from build123d import *

# Parameters (mm, degrees)
F0_W     = 25
F0_H     = 35
F1_DEPTH = 25
F3_R     = 5


with BuildPart() as f1:
    # F0 (on Top) → F1 (new body)
    with BuildSketch(Plane.XY):
        with Locations((-81.198196, -25.874247)):
            Rectangle(F0_W, F0_H)
        with Locations((-81.198196, 214.125753)):
            Rectangle(F0_W, F0_H)
        Polygon((-2.448196, 256.625753), (-68.698196, 256.625753), (-68.698196, 231.625753), (-68.698196, 196.625753), (-68.698196, -8.374247), (-68.698196, -43.374247), (-68.698196, -68.374247), (-2.448196, -68.374247), align=None)
    extrude(amount=F1_DEPTH)

    # F2: F1 across face


with BuildPart() as f1_1:
    add(f1.part)
    add(f1.part.mirror(Plane(origin=(-2.448196, 94.125753, 12.5), x_dir=(0, 1, 0), z_dir=(1, 0, 0))))

    # F3
    f3_edges = [f1_1.edges().sort_by_distance(p)[0] for p in [
        (-2.448196, 256.625753, 0),
        (-2.448196, 256.625753, 25),
        (-2.448196, -68.374247, 0),
        (-2.448196, -68.374247, 25),
    ]]
    fillet(f3_edges, radius=F3_R)


solid = f1_1.part
Design review of the part built by this model. Coordinates are the model's own, in mm. A direction names the side the tool comes from. Coordinates: 2 decimals unless noted, no trailing zeros. Order: outer loops, then holes, each group sorted by start corner. A loop starts at its lowest first (then second) coordinate and runs counter-clockwise, first axis right, second up. Notation, with made-up numbers: (-8, 34) -> (4, 34) arc R10 ccw to (4, 43) -> close; hole circle Ø7 at (-13, 6.5). An arc over 180 degrees is marked (long way). Use one line per item in the form item = value. Start each with the question number.
(1) For faces 5 (the flat face through (-68.698, 244, 12)), 6 (the flat face through (-81, 196.626, 12)), 7 (the flat face through (63.802, 96, 12)), 8 (the flat face through (-68.698, -56, 12)), list the 3-axis set-ups (+Z, -Z, +X, -X, +Y, -Y) from which the entire face can be reached by the end or side of a thin tool; tool diameter is ignored.
(2) The part is to be moulded in two halves that separate along Y. For faces 1 (the flat face through (-1, 96, 25)), 2 (the flat face through (76, -43.374, 12)), 3 (the flat face through (76, 196.626, 12)), 4 (the flat face through (-68.698, 96, 12)), say which applies: +Y half, -Y half, draft (parallel to the pull), parting line (faces both ways), or undercut.
(3) Add section B-B on y = 140. State the section outline as (x, z) points, plus the area to 3 significant figures.
(4) Add section A-A on z = 13.75. State the section outline as (x, y) points, plus the area to 3 significant figures.
(5) Insertion check: pin 1 (12.5 mm diameter, centred on y = 81.5, z = 16.5, fed in from -X); pin 2 (4 mm diameter, centred on y = 171.5, z = 14.5, fed in from +X); pin 3 (10 mm diameter, centred on x = -40.5, z = 4.5, fed in from -Y); pin 4 (7.5 mm diameter, centred on x = 79, z = 14, fed in from +Y). Each pin has a flat end and moves straight along its axis. Give the tip position at first contact, or say it passes through.
(6) For probe 1 along Y at (x, z) = (72, 9); probe 2 along X at (y, z) = (18, 4.5); probe 3 along Y at (x, z) = (-67.5, 4.5), list the stretches that pass through material, from the lowest coordinate up.
Answer block:
q1.face_5 = +Z, -Z, -X, +Y
q1.face_6 = +Z, -Z, -X
q1.face_7 = +Z, -Z, +X
q1.face_8 = +Z, -Z, -X, -Y
q2.face_1 = draft
q2.face_2 = -Y half
q2.face_3 = undercut
q2.face_4 = undercut
q3.outline = (-68.7, 0) -> (63.8, 0) -> (63.8, 25) -> (-68.7, 25) -> close
q3.area = 3,310 mm²
q4.outline = (-93.7, -43.37) -> (-68.7, -43.37) -> (-68.7, -68.37) -> (63.8, -68.37) -> (63.8, -43.37) -> (88.8, -43.37) -> (88.8, -8.37) -> (63.8, -8.37) -> (63.8, 196.63) -> (88.8, 196.63) -> (88.8, 231.63) -> (63.8, 231.63) -> (63.8, 256.63) -> (-68.7, 256.63) -> (-68.7, 231.63) -> (-93.7, 231.63) -> (-93.7, 196.63) -> (-68.7, 196.63) -> (-68.7, -8.37) -> (-93.7, -8.37) -> close
q4.area = 46,600 mm²
q5.pin_1 = -68.7
q5.pin_2 = 63.8
q5.pin_3 = -68.37
q5.pin_4 = 231.63
q6.probe_1 = -43.37 to -8.37, 196.63 to 231.63
q6.probe_2 = -68.7 to 63.8
q6.probe_3 = -68.35 to 256.6
